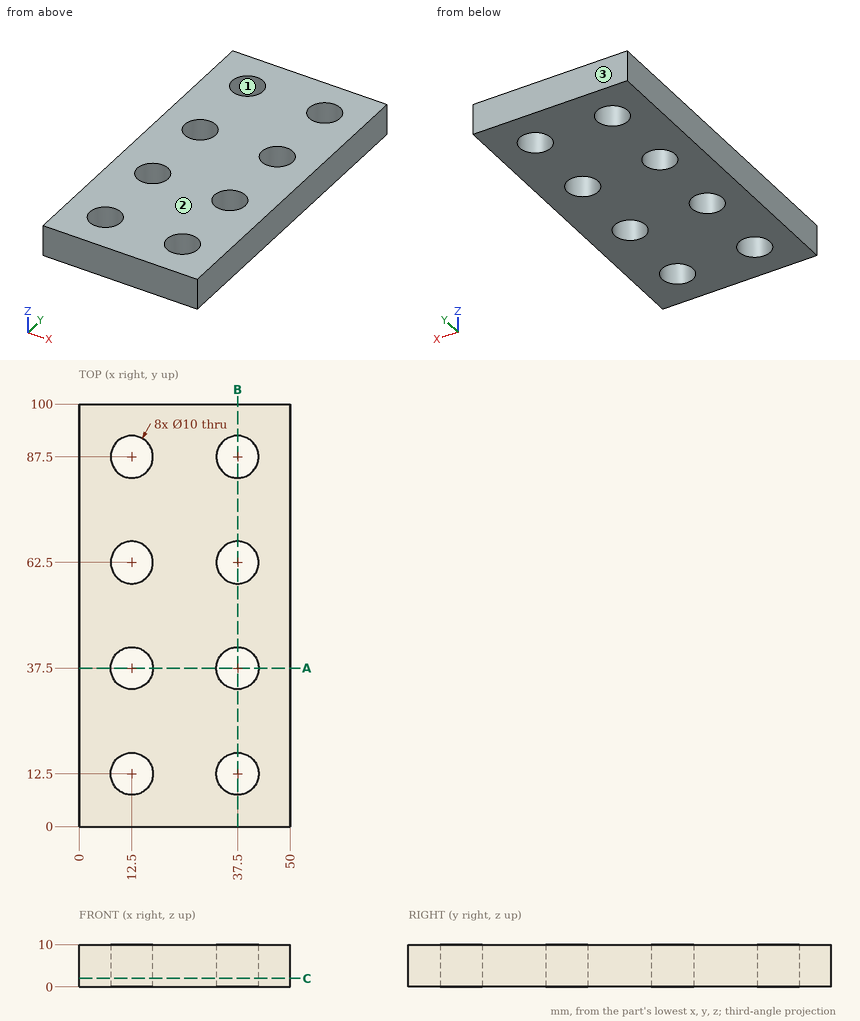
Print and shaded views of the part. All mm, measured from the part's lowest x, y and z. Round coordinates to 2 decimals unless told otherwise and drop trailing zeros. Loops run counter-clockwise (first coordinate to the right, second up) from the corner with the lowest first, then second, coordinate; pieces in that order, holes last. Notation, with made-up numbers: M 9.25,36.25 L 26.25,36.25 A13 cw 26.25,57.25 Z; hole C 72,15.5 d3. An arc over 180 degrees is marked long. One line per question, with ' | ' between items.
1) Band-saw the part on C-C (z = 2). Give the number of separate pieces and of enclosed holes in the cut face, then the cut area to 3 significant figures.
Solved:
separate pieces: 1 | enclosed holes: 8 | area: 4,370 mm²
2) Mould opens along Y. For the marked faces 1, 2 and 3 say: +Y half, -Y half, draft (parallel to the pull), parting line (faces both ways), or undercut.
Solved:
face 1: undercut | face 2: draft | face 3: +Y half
3) Drill centre lines: line 1 along X through (y, z) = (12.5, 6.5); line 2 along Y through (x, z) = (12.5, 5.25); line 3 along Y through (x, z) = (33, 6.25). Where is each one in solid material? Low to high.
Solved:
line 1: x = 0 to 7.5, 17.5 to 32.5, 42.5 to 50 | line 2: y = 0 to 7.5, 17.5 to 32.5, 42.5 to 57.5, 67.5 to 82.5, 92.5 to 100 | line 3: y = 0 to 10.32, 14.68 to 35.32, 39.68 to 60.32, 64.68 to 85.32, 89.68 to 100
4) Band-saw the part on A-A (y = 37.5). Give the cut face in (x, z), then the cut area to 3 significant figures.
Solved:
outline: M 0,0 L 7.5,0 L 7.5,10 L 0,10 Z; M 17.5,0 L 32.5,0 L 32.5,10 L 17.5,10 Z; M 42.5,0 L 50,0 L 50,10 L 42.5,10 Z | area: 300 mm²
5) Band-saw the part on B-B (x = 37.5). Give the cut face in (y, z), then the cut area to 3 significant figures.
Solved:
outline: M 0,0 L 7.5,0 L 7.5,10 L 0,10 Z; M 17.5,0 L 32.5,0 L 32.5,10 L 17.5,10 Z; M 42.5,0 L 57.5,0 L 57.5,10 L 42.5,10 Z; M 67.5,0 L 82.5,0 L 82.5,10 L 67.5,10 Z; M 92.5,0 L 100,0 L 100,10 L 92.5,10 Z | area: 600 mm²
